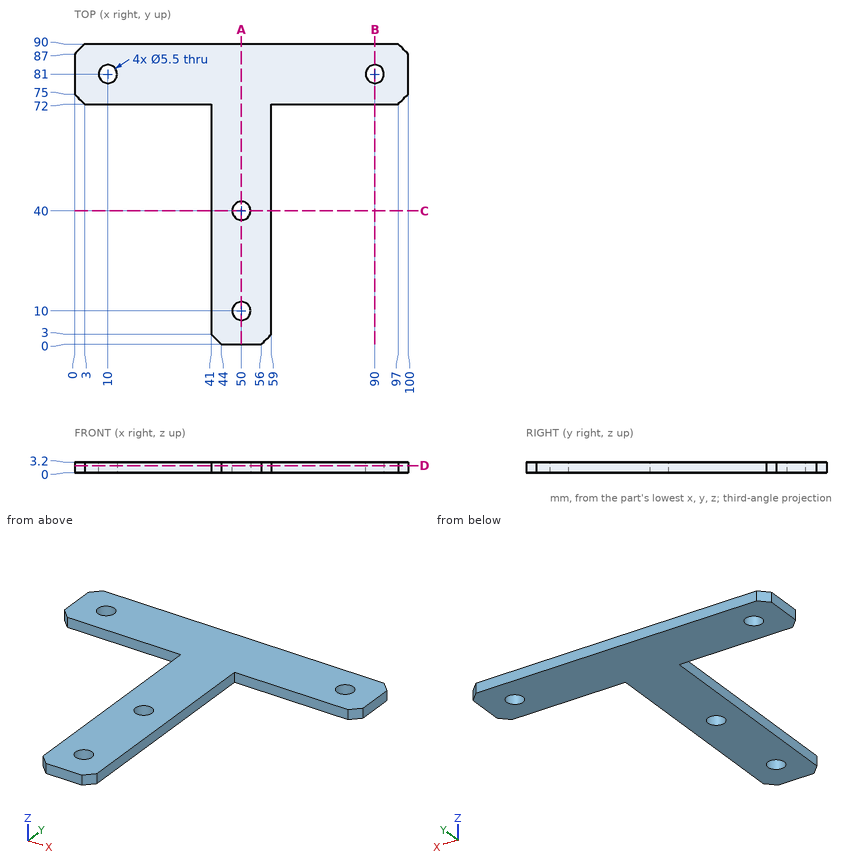
Can you work these out from the drawing? Everything is in mm from the part's minimum corner. Round coordinates to 2 decimals unless told otherwise and drop trailing zeros. Loops run counter-clockwise (first coordinate to the right, second up) from the corner with the lowest first, then second, coordinate; pieces in that order, holes last.
1. If we section it at C-C on y = 40: Write out the boundary of the cut face in (x, z).
Answer list:
outline: (41, 0) - (47.25, 0) - (47.25, 3.2) - (41, 3.2) - close; (52.75, 0) - (59, 0) - (59, 3.2) - (52.75, 3.2) - close
2. If we section it at D-D on z = 2.2: Write out the boundary of the cut face in (x, y).
Answer list:
outline: (0, 75) - (3, 72) - (41, 72) - (41, 3) - (44, 0) - (56, 0) - (59, 3) - (59, 72) - (97, 72) - (100, 75) - (100, 87) - (97, 90) - (3, 90) - (0, 87) - close; hole circle Ø5.5 at (10, 81); hole circle Ø5.5 at (50, 10); hole circle Ø5.5 at (50, 40); hole circle Ø5.5 at (90, 81)
3. For P1, Ø1.6, axis at y = 29.5, z = 1.5, coming from the -X side, with a flat end and sliding along its axis, tell me the tip position at first contact or that it passes through.
Answer list:
P1: stops at x = 41
4. If we section it at B-B on x = 90: Write out the boundary of the cut face in (y, z), plus the area to 3 significant figures.
Answer list:
outline: (72, 0) - (78.25, 0) - (78.25, 3.2) - (72, 3.2) - close; (83.75, 0) - (90, 0) - (90, 3.2) - (83.75, 3.2) - close
area: 40.0 mm2
5. If I drill on line 1 along Y through (x, z) = (50, 1.5); line 2 along Y through (x, z) = (90, 2.2); line 3 along Y through (x, z) = (52, 1.5), over which ranges is the centre line in solid material (lowest first)?
Answer list:
line 1: y = 0 to 7.25, 12.75 to 37.25, 42.75 to 90
line 2: y = 72 to 78.25, 83.75 to 90
line 3: y = 0 to 8.11, 11.89 to 38.11, 41.89 to 90
6. If we section it at A-A on x = 50: Write out the boundary of the cut face in (y, z), plus the area to 3 significant figures.
Answer list:
outline: (0, 0) - (7.25, 0) - (7.25, 3.2) - (0, 3.2) - close; (12.75, 0) - (37.25, 0) - (37.25, 3.2) - (12.75, 3.2) - close; (42.75, 0) - (90, 0) - (90, 3.2) - (42.75, 3.2) - close
area: 253 mm2
